```python
from build123d import *

# Parameters (mm, degrees)
F1_DEPTH = 15
F2_DEPTH = 13
F3_DEPTH = 10.5
F4_DEPTH = 10.5
F6_DEPTH = 30


with BuildPart() as f1:
    # F0 (on Right) → F1 (new body, symmetric)
    with BuildSketch(Plane.YZ):
        Polygon((-24.5765640131, 26.311393382), (-15, 0), (-12.871644455, 0), (-14.0529973008, 3.2457402682), (-22.4482084682, 26.311393382), align=None)
        Polygon((-22.4482084682, 26.311393382), (-14.0529973008, 3.2457402682), (-12.6434583696, 3.7587704831), (-20.8519418095, 26.311393382), align=None)
        Polygon((-14.0529973008, 3.2457402682), (-12.871644455, 0), (-11.2753777963, 0), (-12.6434583696, 3.7587704831), align=None)
        Polygon((-12.6434583696, 3.7587704831), (-11.2753777963, 0), (15, 0), (15, 26.311393382), (-20.8519418095, 26.311393382), align=None)
    extrude(amount=F1_DEPTH, both=True)

    # F0 (on Right) → F2 (cut, symmetric)
    with BuildSketch(Plane.YZ):
        Polygon((-22.4482084682, 26.311393382), (-14.0529973008, 3.2457402682), (-12.6434583696, 3.7587704831), (-20.8519418095, 26.311393382), align=None)
    extrude(amount=F2_DEPTH, both=True, mode=Mode.SUBTRACT)

    # F0 (on Right) → F3 (cut, symmetric)
    with BuildSketch(Plane.YZ):
        Polygon((-24.5765640131, 26.311393382), (-15, 0), (-12.871644455, 0), (-14.0529973008, 3.2457402682), (-22.4482084682, 26.311393382), align=None)
    extrude(amount=F3_DEPTH, both=True, mode=Mode.SUBTRACT)

    # F0 (on Right) → F4 (cut, symmetric)
    with BuildSketch(Plane.YZ):
        Polygon((-14.0529973008, 3.2457402682), (-12.871644455, 0), (-11.2753777963, 0), (-12.6434583696, 3.7587704831), align=None)
    extrude(amount=F4_DEPTH, both=True, mode=Mode.SUBTRACT)

    # F5 (on face) → F6 (cut)
    with BuildSketch(Plane(origin=(0, 0, 0), x_dir=(1, 0, 0), z_dir=(0, 0, -1))):
        Polygon((0, -5), (-15, 10), (-15, -15), (15, -15), (15, 10), align=None)
    extrude(amount=-F6_DEPTH, mode=Mode.SUBTRACT)


solid = f1.part
```
The listing builds one solid part. Answer for the finished solid, in the listing's coordinates (mm). A direction names the side the tool comes from. Give positions to 0.01 mm unless a question says otherwise; leave off trailing zeros. Order: outer loops, then holes, each group sorted by start corner. A loop starts at its lowest first (then second) coordinate and runs counter-clockwise, first axis right, second up. Notation, with made-up numbers: (79.5, 49) -> (126.5, 49) arc R18 cw to (126.5, 53) -> close; hole circle Ø6 at (35, 43). An arc over 180 degrees is marked (long way). Write each question's results on one line, items separated by ' | '.
Q1. Straight lines are drawn through the part: probe 1 along X at (y, z) = (-21.5, 18); probe 2 along Y at (x, z) = (9.5, 1.5); probe 3 along Y at (x, z) = (-9.5, 9). For each, find the intervals that lie inside material, in ascending order. Write a range as from..to.
Checked values:
probe 1: x = -15..-10.5, 10.5..15 | probe 2: y = -11.82..-4.5 | probe 3: y = -14.55..-4.5
Q2. The part is cut by section A-A, the plane x = 12. Give the vertices of the cut face in (y, z), and give its area (3 significant figures).
Checked values:
outline: (-24.58, 26.31) -> (-15, 0) -> (-7, 0) -> (-7, 26.31) -> (-20.85, 26.31) -> (-12.64, 3.76) -> (-14.05, 3.25) -> (-22.45, 26.31) -> close | area: 300 mm^2
Q3. The part is cut by section B-B, the plane z = 19.5. Give the vertices of the cut face in (x, y).
Checked values:
outline: (-15, -22.1) -> (-10.5, -22.1) -> (-10.5, -19.97) -> (-13, -19.97) -> (-13, -18.37) -> (13, -18.37) -> (13, -19.97) -> (10.5, -19.97) -> (10.5, -22.1) -> (15, -22.1) -> (15, -10) -> (0, 5) -> (-15, -10) -> close
Q4. Determine the mould class of faces 4 (the face through (0, -5, 0)), 5 (the face through (-12.718, -19.855, 13.34)), 6 (the face through (-11.73, -18.31, 14.94)) for opening direction Y: pulls with the +Y half, pulls with the -Y half, needs draft (parallel to the pull), parting line crosses it, or undercut.
Checked values:
face 4: needs draft | face 5: pulls with the -Y half | face 6: undercut
Q5. Which of the six approach directions +Z, -Z, +X, -X, +Y, -Y give full straight-line access (tool end or side, diameter ignored) to faces 1 (the face through (0, -13, 26.311)), 2 (the face through (-11.73, -13.36, 3.5)), 3 (the face through (-10.5, -18, 12))?
Checked values:
face 1: +Z, +X, -X, +Y, -Y | face 2: none | face 3: -Z, -Y
Q6. The part is cut by section D-D, the plane x = -5.5. Give the vertices of the cut face in (y, z), and give its area (3 significant figures).
Checked values:
outline: (-20.85, 26.31) -> (-11.28, 0) -> (-0.5, 0) -> (-0.5, 26.31) -> close | area: 410 mm^2
Q7. Each of these flat-tipped pins is pushed along its axis until it touches: P1, Ø8, axis at y = -18.5, z = 9.5, coming from the +X side; P2, Ø8, axis at x = 11.5, y = 1.5, coming from the -Z side; P3, Ø5, axis at x = 11, z = 6, coming from the -Y side; P4, Ø1, axis at y = -4.5, z = 17, coming from the -X side. Where does it stop, or does it pass through?
Checked values:
P1: stops at x = 15 | P2: passes through | P3: stops at y = -18.09 | P4: stops at x = -10
Q8. The part is cut by section C-C, the plane y = 1.25. Give the vertices of the cut face in (x, z).
Checked values:
outline: (-3.75, 0) -> (3.75, 0) -> (3.75, 26.31) -> (-3.75, 26.31) -> close
